Verification items for the finished model (mm, model axes). A direction names the side the tool comes from. Round coordinates to 2 decimals unless told otherwise and drop trailing zeros. Write each loop counter-clockwise with the first axis right and the second up, starting at its lowest first coordinate (ties: lowest second). Pieces come first, ordered by that corner, then holes. Notation, with made-up numbers: M -37.5,-7.5 L 11.5,-7.5 A12 ccw 11.5,2.5 Z; hole C 50.25,5.5 d10. An arc over 180 degrees is marked long. Answer in a Markdown table with one row per item. Add a question column.
1. Sectioned sample at C-C on y = -0.7. Record the cut outline in (x, z).
2. Material ranges on probe 1 along Z at (x, y) = (29.5, -1.05); probe 2 along X at (y, z) = (-1.2, -33.5); probe 3 along X at (y, z) = (1.4, 36.5), recorded low to high.
3. Sectioned sample at A-A on x = -16. Record the cut outline in (y, z).
4. Draft check along Z on faces 4 (the cylindrical face through (-93.85, 0.04, -93.93)), 5 (the flat face through (-61, 0, 98)), 6 (the cylindrical face through (-16.9, 0, 77.6)). Enter one of: pulls with the +Z half, pulls with the -Z half, needs draft (parallel to the pull), parting line crosses it, or undercut.
5. Sectioned sample at D-D on x = 49. Record the cut outline in (y, z).
6. Set-up check for faces 1 (the flat face through (-76, 0, 95.5)), 2 (the flat face through (29, 0, 98)), 3 (the flat face through (-74, 0, -19)): record each of +Z, -Z, +X, -X, +Y, -Y from which the full face is reachable in a straight line by a thin tool's end or side.
7. Go/stop test with a flat-tipped pin: pin 1 Ø2.5 at (y, z) = (0.5, 99.5) entering from +X. Record where the tip stops, or that it passes through.
8. Sectioned sample at B-B on z = -40.5. Record the cut outline in (x, y), plus the area to 3 significant figures.
```python
from build123d import *

# Parameters (mm, degrees)
BOSS_EXTRUDE1_DEPTH = 2.5
CUT_EXTRUDE1_DEPTH  = 6
SKETCH3_W           = 90
SKETCH3_H           = 5.5
BOSS_EXTRUDE2_DEPTH = 5


with BuildPart() as part:
    # Sketch1 → Boss-Extrude1 (new body, symmetric)
    with BuildSketch(Plane(origin=(0, 0, 0), x_dir=(1, 0, 0), z_dir=(0, 1, 0))):
        with BuildLine():
            Line((90, 95.5), (-90, 95.5))
            ThreePointArc((-90, 95.5), (-93.889087297, 93.889087297), (-95.5, 90))
            Line((-95.5, 90), (-95.5, -90))
            ThreePointArc((-95.5, -90), (-93.889087297, -93.889087297), (-90, -95.5))
            Line((-90, -95.5), (90, -95.5))
            ThreePointArc((90, -95.5), (93.889087297, -93.889087297), (95.5, -90))
            Line((95.5, -90), (95.5, 90))
            ThreePointArc((95.5, 90), (93.889087297, 93.889087297), (90, 95.5))
        make_face()
    extrude(amount=BOSS_EXTRUDE1_DEPTH, both=True)

    # Sketch2 → Cut-Extrude1 (cut, through all)
    with BuildSketch(Plane(origin=(0, 2.5, 0), x_dir=(1, 0, 0), z_dir=(0, 1, 0))):
        with BuildLine():
            Line((42, 71), (-74, 71))
            Line((-74, 71), (-74, -34.610229671))
            Line((-74, -34.610229671), (-59, -34.610229671))
            ThreePointArc((-59, -34.610229671), (-16, -77.610229671), (27, -34.610229671))
            Line((27, -34.610229671), (42, -34.610229671))
            Line((42, -34.610229671), (42, 71))
        make_face()
    extrude(amount=-CUT_EXTRUDE1_DEPTH, mode=Mode.SUBTRACT)

    # Sketch3 → Boss-Extrude2 (add)
    with BuildSketch(Plane(origin=(0, 2.5, 0), x_dir=(1, 0, 0), z_dir=(0, 1, 0))):
        with Locations((-16, -98.25)):
            Rectangle(SKETCH3_W, SKETCH3_H)
    extrude(amount=-BOSS_EXTRUDE2_DEPTH)


solid = part.part
```
Geometry check:
| question | item | result |
|---|---|---|
| 1 | outline | M -95.5,-90 A5.5 ccw -90,-95.5 L 90,-95.5 A5.5 ccw 95.5,-90 L 95.5,90 A5.5 ccw 90,95.5 L 29,95.5 L 29,101 L -61,101 L -61,95.5 L -90,95.5 A5.5 ccw -95.5,90 Z; hole M -74,-71 L 42,-71 L 42,34.61 L 27,34.61 A43 ccw -59,34.61 L -74,34.61 Z |
| 2 | probe 1 | z = -95.5 to -71, 34.61 to 95.5 |
| 2 | probe 2 | x = -95.5 to -74, 42 to 95.5 |
| 2 | probe 3 | x = -95.5 to -58.96, 26.96 to 95.5 |
| 3 | outline | M -2.5,-95.5 L 2.5,-95.5 L 2.5,-71 L -2.5,-71 Z; M -2.5,77.61 L 2.5,77.61 L 2.5,101 L -2.5,101 Z |
| 4 | face 4 | pulls with the -Z half |
| 4 | face 5 | needs draft |
| 4 | face 6 | undercut |
| 5 | outline | M -2.5,-95.5 L 2.5,-95.5 L 2.5,95.5 L -2.5,95.5 Z |
| 6 | face 1 | +Z, -X, +Y, -Y |
| 6 | face 2 | +Z, +X, +Y, -Y |
| 6 | face 3 | +Y, -Y |
| 7 | pin 1 | stops at x = 29 |
| 8 | outline | M -95.5,-2.5 L -74,-2.5 L -74,2.5 L -95.5,2.5 Z; M 42,-2.5 L 95.5,-2.5 L 95.5,2.5 L 42,2.5 Z |
| 8 | area | 375 mm2 |
